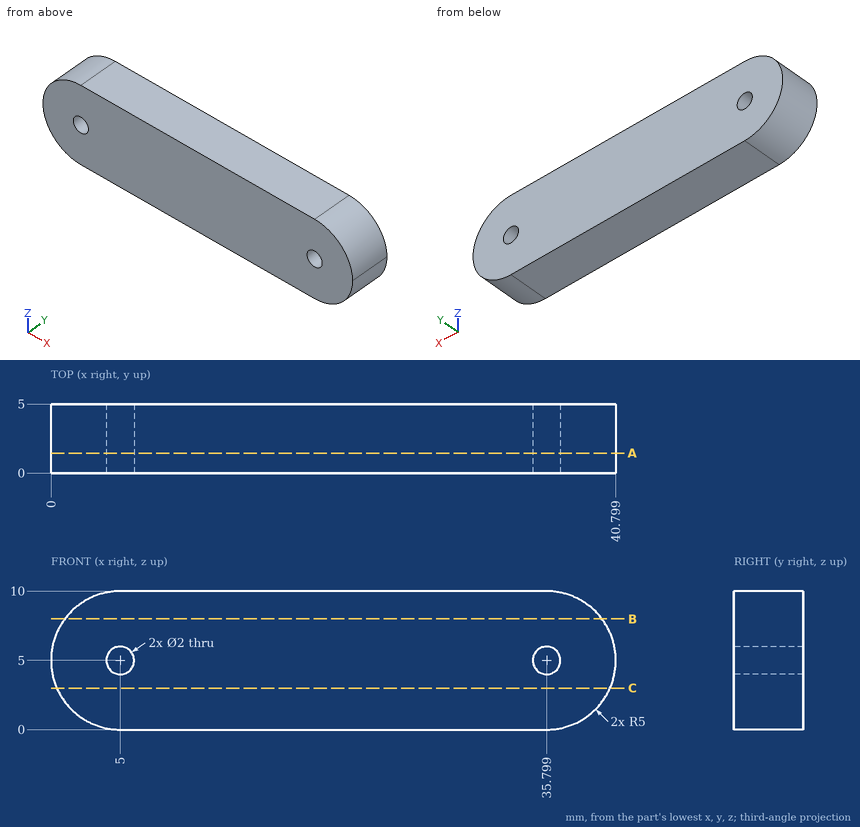
Source: three-view drawing plus pictorial views. Frame: mm from the lowest corner of the part. Round coordinates to 2 decimals unless told otherwise and drop trailing zeros. Order: outer loops, then holes, each group sorted by start corner. A loop starts at its lowest first (then second) coordinate and runs counter-clockwise, first axis right, second up. Notation, with made-up numbers: (86.25, 41) -> (114.25, 41) arc R13 cw to (114.25, 53) -> close; hole circle Ø3 at (59.5, -29). An arc over 180 degrees is marked (long way). Use one line per item in the form item = value.
(1) Section A-A on y = 1.45. Return loops of the section in (x, z), and give its area (3 significant figures).
Results list:
outline = (5, 0) -> (35.8, 0) arc R5 ccw to (35.8, 10) -> (5, 10) arc R5 ccw to start; hole circle Ø2 at (5, 5); hole circle Ø2 at (35.8, 5)
area = 380 mm^2
(2) Section C-C on z = 3. Return loops of the section in (x, y).
Results list:
outline = (0.42, 0) -> (40.38, 0) -> (40.38, 5) -> (0.42, 5) -> close
(3) Ray query, probe 1 along X at (y, z) = (2.45, 5); probe 2 along Z at (x, y) = (5, 2.1); probe 3 along X at (y, z) = (1.6, 4.5) (1 decimal). Return the intervals inside material, ascending. Write a range as [from, to].
Results list:
probe_1 = [0, 4], [6, 34.8], [36.8, 40.8]
probe_2 = [0, 4], [6, 10]
probe_3 = [0, 4.1], [5.9, 34.9], [36.7, 40.8]
(4) First-contact query: pin 1 Ø1.8 at (x, z) = (35.8, 5) entering from +Y; pin 2 Ø6 at (x, z) = (10.5, 2.5) entering from -Y; pin 3 Ø3 at (y, z) = (3, 1.5) entering from +X. Flat tips, straight axial feed; report the tip coordinate or a pass-through.
Results list:
pin_1 = through
pin_2 = 0
pin_3 = 40.38
(5) Section B-B on z = 8. Return loops of the section in (x, y).
Results list:
outline = (1, 0) -> (39.8, 0) -> (39.8, 5) -> (1, 5) -> close
